```python
from build123d import *

# Parameters (mm, degrees)
SKETCH1_W           = 270
SKETCH1_H           = 110
BOSS_EXTRUDE1_DEPTH = 4
SKETCH9_R           = 3
CUT_EXTRUDE1_DEPTH  = 146.828666592
SKETCH10_W          = 270
SKETCH10_H          = 4
BOSS_EXTRUDE2_DEPTH = 30
ESQUISSE1_W         = 4
ESQUISSE1_H         = 28
BOSS_EXTRU_1_DEPTH  = 5


with BuildPart() as part:
    # Sketch1 → Boss-Extrude1 (new body)
    with BuildSketch(Plane.XY):
        Rectangle(SKETCH1_W, SKETCH1_H)
    extrude(amount=BOSS_EXTRUDE1_DEPTH)

    # Sketch9 → Cut-Extrude1 (cut, through all)
    with BuildSketch(Plane(origin=(0, 0, 0), x_dir=(-1, 0, 0), z_dir=(0, 0, -1))):
        with Locations((-120, 46)):
            Circle(SKETCH9_R)
        with Locations((-127, -46)):
            Circle(SKETCH9_R)
        with Locations((120, 46)):
            Circle(SKETCH9_R)
        with Locations((127, -46)):
            Circle(SKETCH9_R)
    extrude(amount=-CUT_EXTRUDE1_DEPTH, mode=Mode.SUBTRACT)

    # Sketch10 → Boss-Extrude2 (add)
    with BuildSketch(Plane(origin=(0, 55, 0), x_dir=(1, 0, 0), z_dir=(0, 1, 0))):
        with Locations((0, -2)):
            Rectangle(SKETCH10_W, SKETCH10_H)
    extrude(amount=BOSS_EXTRUDE2_DEPTH)

    # Esquisse1 → Boss.-Extru.1 (add)
    with BuildSketch(Plane(origin=(135, 0, 0), x_dir=(0, 0, -1), z_dir=(1, 0, 0))):
        with Locations((-2, -13)):
            Rectangle(ESQUISSE1_W, ESQUISSE1_H)
        with Locations((-2, 43)):
            Rectangle(ESQUISSE1_W, ESQUISSE1_H)
    boss_extru_1 = extrude(amount=BOSS_EXTRU_1_DEPTH)

    # Symétrie1: Boss.-Extru.1 across plane
    add(boss_extru_1.mirror(Plane(origin=(0, 0, 0), x_dir=(0, 0, 1), z_dir=(1, 0, 0))))


solid = part.part
```
Could you check a few things on this model? Use its own coordinates, in mm. Round coordinates to 2 decimals unless told otherwise and drop trailing zeros. Write each loop counter-clockwise with the first axis right and the second up, starting at its lowest first coordinate (ties: lowest second). Pieces come first, ordered by that corner, then holes.
(1) Thinking about a two-plate mould opening in X: for faces 1 (the face through (-122.86, 46.9, 1.97)), 2 (the face through (-2, 14, 4)), which applies, +X half, -X half, draft (parallel to the pull), parting line (faces both ways), or undercut?
Findings below:
face 1: undercut
face 2: draft
(2) Suppose I cut it at D-D on y = 67. Write out the boundary of the cut face in (x, z), and give its area (3 significant figures).
Findings below:
outline: (-135, 0) - (135, 0) - (135, 4) - (-135, 4) - close
area: 1,080 mm2
(3) If I drill on probe 1 along Y at (x, z) = (119.5, 0.75); probe 2 along Y at (x, z) = (-127, 2.4); probe 3 along X at (y, z) = (78, 2.55), over which ranges is the centre line in solid material (lowest first)?
Findings below:
probe 1: y = -55 to 43.04, 48.96 to 85
probe 2: y = -55 to -49, -43 to 85
probe 3: x = -135 to 135
(4) Suppose I cut it at A-A on y = -46. Write out the boundary of the cut face in (x, z), and give its area (3 significant figures).
Findings below:
outline: (-135, 0) - (-130, 0) - (-130, 4) - (-135, 4) - close; (-124, 0) - (124, 0) - (124, 4) - (-124, 4) - close; (130, 0) - (135, 0) - (135, 4) - (130, 4) - close
area: 1,030 mm2
(5) Suppose I cut it at C-C on z = 1.35. Write out the boundary of the cut face in (x, y), and give its area (3 significant figures).
Findings below:
outline: (-140, -27) - (-135, -27) - (-135, -55) - (135, -55) - (135, -27) - (140, -27) - (140, 1) - (135, 1) - (135, 29) - (140, 29) - (140, 57) - (135, 57) - (135, 85) - (-135, 85) - (-135, 57) - (-140, 57) - (-140, 29) - (-135, 29) - (-135, 1) - (-140, 1) - close; hole circle Ø6 at (-127, -46); hole circle Ø6 at (-120, 46); hole circle Ø6 at (120, 46); hole circle Ø6 at (127, -46)
area: 38,200 mm2
(6) Suppose I cut it at B-B on x = 127. Write out the boundary of the cut face in (y, z), and give its area (3 significant figures).
Findings below:
outline: (-55, 0) - (-49, 0) - (-49, 4) - (-55, 4) - close; (-43, 0) - (85, 0) - (85, 4) - (-43, 4) - close
area: 536 mm2
(7) For pin 1 (5 mm diameter, centred on x = 127, y = -46, fed in from +Z); pin 2 (1.2 mm diameter, centred on y = 77, z = 2.5, fed in from +X); pin 3 (2 mm diameter, centred on y = -40.5, z = 2.5, fed in from -X); pin 4 (10 mm diameter, centred on x = -38.5, y = 31, fed in from -Z), each with a flat end and sliding along its axis, tell me the tip position at first contact or that it passes through.
Findings below:
pin 1: passes through
pin 2: stops at x = 135
pin 3: stops at x = -135
pin 4: stops at z = 0
